from build123d import *

# Parameters (mm, degrees)
SKETCH2_R                   = 2.5
BOSS_EXTRUDE1_DEPTH         = 3
BOSS_EXTRUDE2_START         = 2.75
SKETCH3_W                   = 15
SKETCH3_H                   = 10
BOSS_EXTRUDE2_DEPTH         = 2.5
FILLET2_RADIUS              = 5
FILLET2_LENGTH              = 2.5
FILLET2_OF_MIRROR1_2_RADIUS = 5
FILLET2_OF_MIRROR1_2_LENGTH = 2.5
CHAMFER1_SIZE               = 2
CHAMFER2_SIZE               = 2
SKETCH5_R                   = 2.5
CUT_EXTRUDE2_DEPTH          = 97.675035557
CHAMFER3_SIZE               = 3
FILLET3_R                   = 2.5
CHAMFER4_SIZE               = 1


with BuildPart() as part:
    # Sketch2 → Boss-Extrude1 (new body)
    with BuildSketch(Plane(origin=(0, 0, 0), x_dir=(1, 0, 0), z_dir=(0, 1, 0))):
        Polygon((15, 0), (-15, 0), (-15, -12), (-5, -12), (-5, -82), (-15, -82), (-15, -94), (15, -94), (15, -82), (5, -82), (5, -12), (15, -12), align=None)
        with Locations(Location((-9, -6, 0), (0, 0, 270))):
            Circle(SKETCH2_R, mode=Mode.SUBTRACT)
        with Locations(Location((-9, -88, 0), (0, 0, 270))):
            Circle(SKETCH2_R, mode=Mode.SUBTRACT)
        with Locations(Location((9, -88, 0), (0, 0, 270))):
            Circle(SKETCH2_R, mode=Mode.SUBTRACT)
        with Locations(Location((9, -6, 0), (0, 0, 270))):
            Circle(SKETCH2_R, mode=Mode.SUBTRACT)
    extrude(amount=BOSS_EXTRUDE1_DEPTH)

    # Sketch3 → Boss-Extrude2 (add)
    with BuildSketch(Plane(origin=(0, 0, 0), x_dir=(0, 0, -1), z_dir=(1, 0, 0)).offset(BOSS_EXTRUDE2_START)):
        with Locations((7.5, 5)):
            Rectangle(SKETCH3_W, SKETCH3_H)
    boss_extrude2 = extrude(amount=BOSS_EXTRUDE2_DEPTH)

    # Fillet2: full round fillet: the end face becomes a half cylinder, R = half its width
    fillet2_face = Plane((4, 5, -15), x_dir=(-1, 0, 0), z_dir=(0, 0, -1))  # on the end face: x along it, z out of the body
    fillet2_slab = fillet2_face.offset(-FILLET2_RADIUS / 2) * Box(FILLET2_LENGTH, 2 * FILLET2_RADIUS, FILLET2_RADIUS, mode=Mode.PRIVATE)  # the body's end, R deep
    fillet2_round = Plane((4, 5, -10), x_dir=(0, 0, -1), z_dir=(-1, 0, 0)) * Cylinder(FILLET2_RADIUS, FILLET2_LENGTH, mode=Mode.PRIVATE)  # its axis R under the face
    add(fillet2_slab - fillet2_round, mode=Mode.SUBTRACT)

    # Mirror1: Boss-Extrude2 across plane
    add(boss_extrude2.mirror(Plane(origin=(0, 0, 0), x_dir=(0, 0, 1), z_dir=(1, 0, 0))))

    # Fillet2 of Mirror1 2: full round fillet: the end face becomes a half cylinder, R = half its width
    fillet2_of_mirror1_2_face = Plane((-4, 5, -15), x_dir=(1, 0, 0), z_dir=(0, 0, -1))  # on the end face: x along it, z out of the body
    fillet2_of_mirror1_2_slab = fillet2_of_mirror1_2_face.offset(-FILLET2_OF_MIRROR1_2_RADIUS / 2) * Box(FILLET2_OF_MIRROR1_2_LENGTH, 2 * FILLET2_OF_MIRROR1_2_RADIUS, FILLET2_OF_MIRROR1_2_RADIUS, mode=Mode.PRIVATE)  # the body's end, R deep
    fillet2_of_mirror1_2_round = Plane((-4, 5, -10), x_dir=(0, 0, -1), z_dir=(1, 0, 0)) * Cylinder(FILLET2_OF_MIRROR1_2_RADIUS, FILLET2_OF_MIRROR1_2_LENGTH, mode=Mode.PRIVATE)  # its axis R under the face
    add(fillet2_of_mirror1_2_slab - fillet2_of_mirror1_2_round, mode=Mode.SUBTRACT)

    # Chamfer1
    chamfer1_edges = [part.edges().sort_by_distance(p)[0] for p in [
        (4, 3, 0),
        (-4, 3, 0),
    ]]
    chamfer(chamfer1_edges, length=CHAMFER1_SIZE)

    # Chamfer2
    chamfer2_edges = [part.edges().sort_by_distance(p)[0] for p in [
        (-5.25, 1.5, 0),
        (5.25, 1.5, 0),
        (4, 10, 0),
        (-4, 10, 0),
    ]]
    chamfer(chamfer2_edges, length=CHAMFER2_SIZE)

    # Sketch5 → Cut-Extrude2 (cut, through all)
    with BuildSketch(Plane(origin=(5.25, 0, 0), x_dir=(0, 0, -1), z_dir=(1, 0, 0))):
        with Locations((10, 5)):
            Circle(SKETCH5_R)
    extrude(amount=-CUT_EXTRUDE2_DEPTH, mode=Mode.SUBTRACT)

    # Chamfer3
    chamfer3_edges = [part.edges().sort_by_distance(p)[0] for p in [
        (15, 1.5, 12),
        (5, 1.5, 12),
        (5, 1.5, 82),
        (15, 1.5, 82),
        (15, 1.5, 94),
        (-15, 1.5, 94),
        (-15, 1.5, 82),
        (-5, 1.5, 82),
        (-5, 1.5, 12),
        (-15, 1.5, 12),
        (-15, 1.5, 0),
        (15, 1.5, 0),
    ]]
    chamfer(chamfer3_edges, length=CHAMFER3_SIZE)

    # Fillet3
    fillet3_edges = [part.edges().sort_by_distance(p)[0] for p in [
        (-15, 1.5, 85),
        (-12, 1.5, 82),
        (-8, 1.5, 82),
        (-5, 1.5, 79),
        (-5, 1.5, 15),
        (-8, 1.5, 12),
        (-12, 1.5, 12),
        (-15, 1.5, 9),
        (-12, 1.5, 0),
        (-7.25, 1.5, 0),
        (-5.25, 1.5, -2),
        (-2.75, 1.5, 0),
        (2.75, 1.5, 0),
        (5.25, 1.5, -2),
        (7.25, 1.5, 0),
        (12, 1.5, 0),
        (15, 1.5, 3),
        (15, 1.5, 9),
        (12, 1.5, 12),
        (8, 1.5, 12),
        (5, 1.5, 15),
        (5, 1.5, 79),
        (8, 1.5, 82),
        (12, 1.5, 82),
        (15, 1.5, 85),
        (15, 1.5, 91),
        (12, 1.5, 94),
        (-12, 1.5, 94),
        (-15, 1.5, 91),
        (-15, 1.5, 3),
        (4, 8, 0),
        (4, 10, -2),
        (-4, 10, -2),
        (-4, 8, 0),
    ]]
    fillet(fillet3_edges, radius=FILLET3_R)

    # Chamfer4
    chamfer4_edges = [part.edges().sort_by_distance(p)[0] for p in [
        (9, 3, 85.5),
        (-9, 3, 85.5),
        (-9, 3, 3.5),
        (9, 3, 3.5),
    ]]
    chamfer(chamfer4_edges, length=CHAMFER4_SIZE)


solid = part.part
Read the model definition and answer for the solid it produces. Units are mm, in the model's axes. A direction names the side the tool comes from. Give positions to 0.01 mm unless a question says otherwise; leave off trailing zeros. Write each loop counter-clockwise with the first axis right and the second up, starting at its lowest first coordinate (ties: lowest second). Pieces come first, ordered by that corner, then holes. Notation, with made-up numbers: (61.5, 78) - (85.5, 78) arc R21 ccw to (85.5, 115) - close; hole circle Ø9 at (67, 56). An arc over 180 degrees is marked (long way). Answer in a Markdown table with one row per item. Add a question column.
Item 1: Section B-B, the plane z = 21.5 is taken. Write down the section's boundary in (x, y), and give its area (3 significant figures).
Item 2: Determine the mould class of faces 5 (the face through (10, 1, 12)), 6 (the face through (-11.934, 1.521, 82.196)), 7 (the face through (-10.5, 1, 86)) for opening direction X: pulls with the +X half, pulls with the -X half, needs draft (parallel to the pull), parting line crosses it, or undercut.
Item 3: Find the intervals of material crossed by L1, parallel to X at y = 0.95, z = 6; L2, parallel to Y at x = 4.05, z = -10; L3, parallel to X at y = 6.5, z = -5, in increasing order.
Item 4: Section A-A, the plane z = 88 is taken. Write down the section's boundary in (x, y), and give its area (3 significant figures).
Item 5: Flat-ended cylindrical pins translate along their axes: P1, Ø8, axis at x = -9, z = 88, coming from the +Y side; P2, Ø0.9, axis at y = 2, z = 34, coming from the -X side; P3, Ø1, axis at x = -10.5, y = 1.5, coming from the -Z side. Find the tip coordinate at first contact, or state that the pin passes through.
Item 6: A tool of negligible diameter and unlimited length cuts with its end or side. For faces 1 (the face through (-10, 1, 12)), 2 (the face through (10, 1, 0)), 3 (the face through (2.037, 1.521, -0.752)), 4 (the face through (5, 1, 47)), from which of +Z, -Z, +X, -X, +Y, -Y can it reach the whole face along a straight path? Write none if from no direction.
Recorded:
| question | item | result |
|---|---|---|
| 1 | outline | (-5, 0) - (5, 0) - (5, 3) - (-5, 3) - close |
| 1 | area | 30.0 mm2 |
| 2 | face 5 | needs draft |
| 2 | face 6 | pulls with the -X half |
| 2 | face 7 | undercut |
| 3 | L1 | x = -15 to -11.5, -6.5 to 6.5, 11.5 to 15 |
| 3 | L2 | y = 0 to 2.5, 7.5 to 10 |
| 3 | L3 | x = -5.25 to -2.75, 2.75 to 5.25 |
| 4 | outline | (-15, 0) - (-11.5, 0) - (-11.5, 2) - (-12.5, 3) - (-15, 3) - close; (-6.5, 0) - (6.5, 0) - (6.5, 2) - (5.5, 3) - (-5.5, 3) - (-6.5, 2) - close; (11.5, 0) - (15, 0) - (15, 3) - (12.5, 3) - (11.5, 2) - close |
| 4 | area | 58.0 mm2 |
| 5 | P1 | stops at y = 3 |
| 5 | P2 | stops at x = -5 |
| 5 | P3 | stops at z = 0 |
| 6 | face 1 | -X, +Y, -Y |
| 6 | face 2 | -Z, +X, +Y, -Y |
| 6 | face 3 | -Z, +Y, -Y |
| 6 | face 4 | +X, +Y, -Y |
